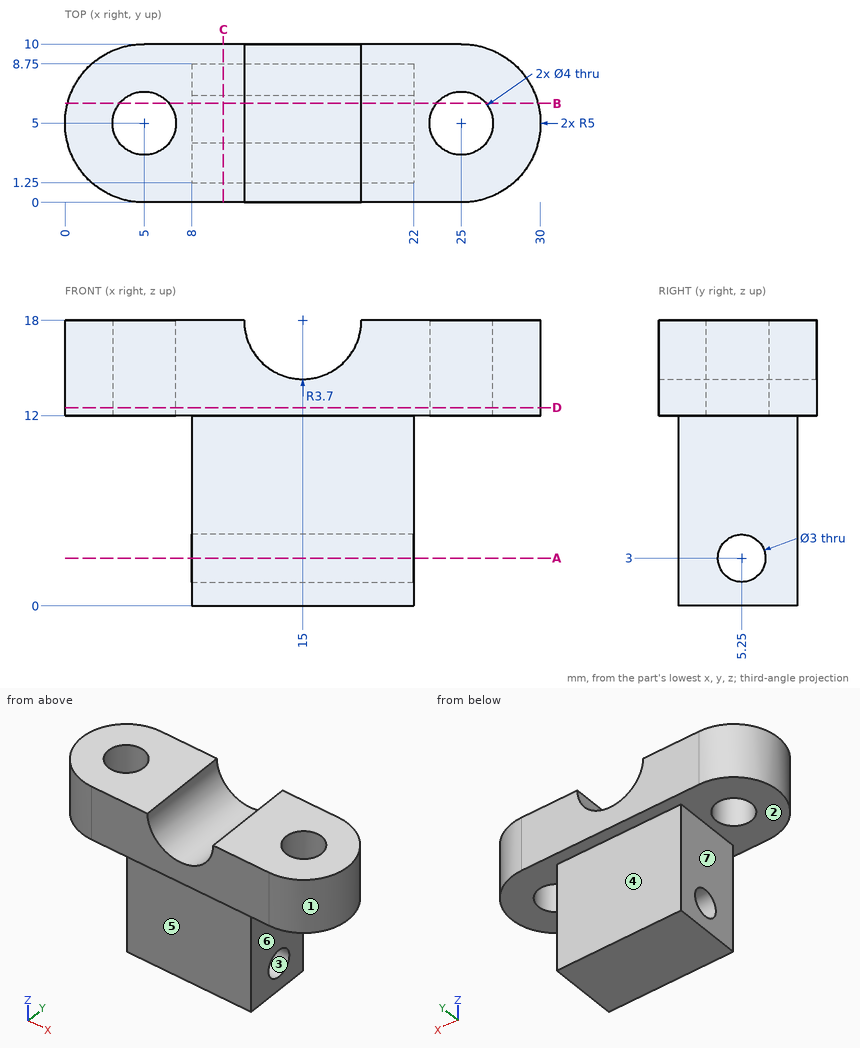
Drawing for the job (mm, zero at the part's lowest x, y, z). A direction names the side the tool comes from. Round coordinates to 2 decimals unless told otherwise and drop trailing zeros. Order: outer loops, then holes, each group sorted by start corner. A loop starts at its lowest first (then second) coordinate and runs counter-clockwise, first axis right, second up.
Item 1: Tool access for the marked faces 5, 6 and 7: list every direction of +Z, -Z, +X, -X, +Y, -Y with a clear straight run to the whole face (end or side of a thin tool).
Item 2: Saw through at C-C on x = 10. Write the cut outline in (y, z), then the cut area to 3 significant figures.
Item 3: Pin check, flat tips, straight feed: pin 1 (3.5 mm diameter, centred on x = 25, y = 5, fed in from -Z); pin 2 (3.5 mm diameter, centred on x = 13.5, z = 4.5, fed in from -Y); pin 3 (4 mm diameter, centred on y = 5.25, z = 3, fed in from -X); pin 4 (3.5 mm diameter, centred on x = 11.5, z = 5.5, fed in from +Y). Stop position of each tip, or through.
Item 4: Saw through at D-D on z = 12.5. Write the cut outline in (x, y).
Item 5: Mould opens along Y. For the marked faces 1, 2, 3 and 4 say: pulls with the +Y half, pulls with the -Y half, needs draft (parallel to the pull), parting line crosses it, or undercut.
Item 6: Saw through at B-B on y = 6.25. Write the cut outline in (x, z).
Item 7: Saw through at A-A on z = 3. Write the cut outline in (x, y), then the cut area to 3 significant figures.
Item 8: Probe line 1 along Y through (x, z) = (5, 13.4); line 2 along X through (y, z) = (6.75, 15.5); line 3 along Y through (x, z) = (14.5, 3). List the from-to ranges inside material, lowest first.
Reported:
1. face 5: -Z, +X, -X, -Y
1. face 6: -Z, +X, +Y, -Y
1. face 7: -Z, -X, +Y, -Y
2. outline: (0, 12) - (1.25, 12) - (1.25, 0) - (8.75, 0) - (8.75, 12) - (10, 12) - (10, 18) - (0, 18) - close; hole circle Ø3 at (5.25, 3)
2. area: 143 mm2
3. pin 1: passes through
3. pin 2: stops at y = 1.25
3. pin 3: stops at x = 8
3. pin 4: stops at y = 8.75
4. outline: (5, 0) - (25, 0) arc R5 ccw to (25, 10) - (5, 10) arc R5 ccw to start; hole circle Ø4 at (5, 5); hole circle Ø4 at (25, 5)
5. face 1: parting line crosses it
5. face 2: needs draft
5. face 3: undercut
5. face 4: pulls with the +Y half
6. outline: (0.16, 12) - (3.44, 12) - (3.44, 18) - (0.16, 18) - close; (6.56, 12) - (8, 12) - (8, 4.12) - (22, 4.12) - (22, 12) - (23.44, 12) - (23.44, 18) - (18.7, 18) arc R3.7 cw to (11.3, 18) - (6.56, 18) - close; (8, 0) - (22, 0) - (22, 1.88) - (8, 1.88) - close; (26.56, 12) - (29.84, 12) - (29.84, 18) - (26.56, 18) - close
7. outline: (8, 1.25) - (22, 1.25) - (22, 3.75) - (8, 3.75) - close; (8, 6.75) - (22, 6.75) - (22, 8.75) - (8, 8.75) - close
7. area: 63.0 mm2
8. line 1: y = 0 to 3, 7 to 10
8. line 2: x = 0.32 to 4.03, 5.97 to 12.27, 17.73 to 24.03, 25.97 to 29.68
8. line 3: y = 1.25 to 3.75, 6.75 to 8.75
